from build123d import *

# Parameters (mm, degrees)
SKETCH_2_W          = 72
SKETCH_2_H          = 72
CUT_EXTRUDE_1_DEPTH = 26


with BuildPart() as part:
    # 草图1 → 旋转1 (revolve)
    with BuildSketch(Plane.XY):
        Polygon((0, 0), (0, 18), (2.078460969, 21.6), (10.921539031, 21.6), (13, 18), (13, 0), align=None)
    revolve(axis=Axis((13, 0, 0), (-1, 0, 0)))

    # 草图2 → 切除-拉伸1 (cut)
    with BuildSketch(Plane(origin=(0, 0, 0), x_dir=(0, 0, -1), z_dir=(1, 0, 0))):
        Rectangle(SKETCH_2_W, SKETCH_2_H)
        Polygon((-18, -10.392304845), (0, -20.784609691), (18, -10.392304845), (18, 10.392304845), (0, 20.784609691), (-18, 10.392304845), align=None, mode=Mode.SUBTRACT)
    extrude(amount=CUT_EXTRUDE_1_DEPTH, mode=Mode.SUBTRACT)

    # 草图3 → 切除-旋转1 (revolve, cut)
    with BuildSketch(Plane.XY):
        Polygon((0, 0), (0, 13), (0.812, 12.188), (12.188, 12.188), (13, 13), (13, 0), align=None)
    revolve(axis=Axis((13, 0, 0), (-1, 0, 0)), mode=Mode.SUBTRACT)


solid = part.part
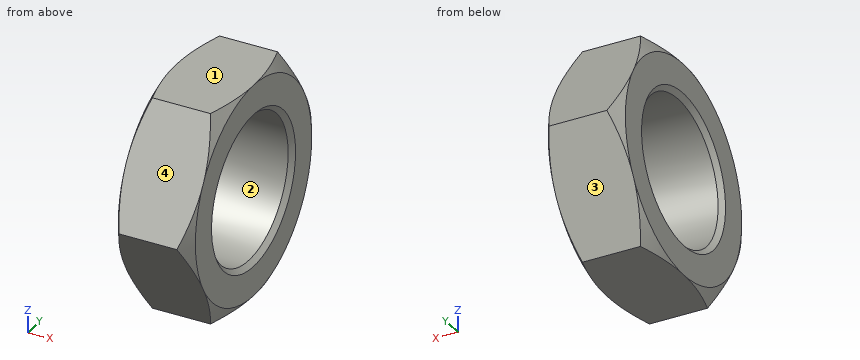
Source: CAD feature listing. Evaluate the final solid. Frame: model axes, mm. Face numbers are marked on the shaded views. Give positions to 0.01 mm unless a question says otherwise; leave off trailing zeros. Write each loop counter-clockwise with the first axis right and the second up, starting at its lowest first coordinate (ties: lowest second). Pieces come first, ordered by that corner, then holes. Notation, with made-up numbers: M 7,-34.5 L 26,-34.5 A27 ccw 26,-2.5 Z; hole C 38,73 d7. An arc over 180 degrees is marked long. Return JSON: item names as keys, results as strings. Group by question number.
1) Cut plane A-A, the plane x = 5.75. Output: boundary loops of the cut face in (y, z).
2) Pin query (flat end, axial travel): P1, Ø1.5, axis at x = 9, z = 14.5, coming from the -Y side; P2, Ø1.5, axis at x = 1.5, z = 13.5, coming from the +Y side. Return the tip coordinate at first contact, or that it passes through.
3) Pull-direction query (Y, two-part tool) for the marked faces 1, 2, 3 and 4; classes: pulls with the +Y half, pulls with the -Y half, needs draft (parallel to the pull), parting line crosses it, or undercut.
4) Material intervals for line 1 along Y through (x, z) = (4.75, 0); line 2 along Z through (x, y) = (3, 10); line 3 along Y through (x, z) = (4.5, 3), sorted ascending. Write a range as [from, to].
Recorded:
{
 "1": {"outline": "M -20.78,0 L -10.39,-18 L 10.39,-18 L 20.78,0 L 10.39,18 L -10.39,18 Z; hole C 0,0 d24.38"},
 "2": {"P1": "stops at y = -12.85", "P2": "stops at y = 13.42"},
 "3": {"face 1": "needs draft", "face 2": "undercut", "face 3": "pulls with the +Y half", "face 4": "pulls with the -Y half"},
 "4": {"line 1": "y = [-20.78, -12.19], [12.19, 20.78]", "line 2": "z = [-18, -6.97], [6.97, 18]", "line 3": "y = [-19.05, -11.81], [11.81, 19.05]"}
}
